Could you check a few things on this model? Use its own coordinates, in mm. A direction names the side the tool comes from. Coordinates: 2 decimals unless noted, no trailing zeros. Loops run counter-clockwise (first coordinate to the right, second up) from the corner with the lowest first, then second, coordinate; pieces in that order, holes last. Notation, with made-up numbers: (40.5, 14) -> (60.5, 14) arc R25 cw to (60.5, 47) -> close; hole circle Ø8 at (13.25, -19.5). An arc over 180 degrees is marked (long way). One line per question, with ' | ' between items. Start each with the question number.
(1) Suppose I cut it at A-A (y = -30.5). Please give me the cut outline in (x, z), plus the area to 3 significant figures.
(2) Which directions (+Z, -Z, +X, -X, +Y, -Y) give clear straight access to the entire face, cutting with the end or side of a thin tool? Please do faces 1 (the face through (33, -5, 2)), 2 (the face through (-28, 9, 2)), 3 (the face through (21.86, -19.44, 4.86)), 4 (the face through (20, 42.1, -1)), 5 (the face through (-32, 2, 0)).
(3) Suppose I cut it at C-C (z = -1). Please give me the cut outline in (x, y), plus the area to 3 significant figures.
(4) If we mould it in two halves opening along X, with no side actions, what happens to faces 6 (the face through (-30, -7, -2)), 7 (the face through (38.997, 0.154, 0.247)), 8 (the face through (28.1, -1, -1))? For each: pulls with the +X half, pulls with the -X half, needs draft (parallel to the pull), parting line crosses it, or undercut.
(5) I'm going to push flat-ended pins straight in: pin 1 Ø2.5 at (x, y) = (-35.5, 0) entering from +Z; pin 2 Ø1 at (y, z) = (40.5, 2.5) entering from +X; pin 3 Ø5 at (x, y) = (-36, 0.5) entering from -Z; pin 4 Ø11 at (x, y) = (-35.5, 0) entering from -Z. Where does each tip first touch, or does it pass through?
(6) If I drill on line 1 along X through (y, z) = (38.5, 1.95); line 2 along Y through (x, z) = (24.5, 3.5); line 3 along Y through (x, z) = (27, 3.75), over which ranges is the centre line in solid material (lowest first)?
(7) Suppose I cut it at D-D (y = 0). Give the number of separate pieces and of enclosed holes in the cut face, plus the area to 3 significant figures.
(8) Suppose I cut it at B-B (x = 6). Please give me the cut outline in (y, z).
```python
from build123d import *
from OCP.BRepFilletAPI import BRepFilletAPI_MakeChamfer

# Parameters (mm, degrees)
SKETCH1_R           = 0.85
BOSS_EXTRUDE1_DEPTH = 5
SKETCH2_W           = 56.2
SKETCH2_H           = 85.2
BOSS_EXTRUDE2_DEPTH = 2
SKETCH3_R           = 2.25
BOSS_EXTRUDE3_DEPTH = 5
SKETCH4_R           = 3.5
CUT_EXTRUDE1_DEPTH  = 3
SKETCH5_W           = 25
SKETCH5_H           = 2.4
CUT_EXTRUDE2_DEPTH  = 62.118736898
CHAMFER3_SIZE       = 0.5
CHAMFER1_SIZE       = 2.5
CHAMFER1_SIZE_2     = 1.25


with BuildPart() as part:
    # Sketch1 → Boss-Extrude1 (new body)
    with BuildSketch(Plane.XY):
        Polygon((-30.5, -43), (-30.5, 44.5), (30.5, 44.5), (30.5, -43), (30.5, -45.5), (-30.5, -45.5), align=None)
        with Locations((-24.5, 38.5)):
            Circle(SKETCH1_R, mode=Mode.SUBTRACT)
        with Locations((24.5, 38.5)):
            Circle(SKETCH1_R, mode=Mode.SUBTRACT)
        with Locations((24.5, -19.5)):
            Circle(SKETCH1_R, mode=Mode.SUBTRACT)
        with Locations((-24.5, -19.5)):
            Circle(SKETCH1_R, mode=Mode.SUBTRACT)
        with BuildLine():
            Line((-21.5, 38.5), (-21.5, 42))
            Line((-21.5, 42), (8, 42))
            Line((8, 42), (8, 35.5))
            Line((8, 35.5), (24.5, 35.5))
            Line((24.5, 35.5), (28, 35.5))
            Line((28, 35.5), (28, -16.5))
            Line((28, -16.5), (24.5, -16.5))
            ThreePointArc((24.5, -16.5), (21.5, -19.5), (24.5, -22.5))
            Line((24.5, -22.5), (28, -22.5))
            Line((28, -22.5), (28, -42))
            Line((28, -42), (5, -42))
            Line((5, -42), (5, -38))
            Line((5, -38), (0, -38))
            Line((0, -38), (-5, -38))
            Line((-5, -38), (-5, -42))
            Line((-5, -42), (-28, -42))
            Line((-28, -42), (-28, -22.5))
            Line((-28, -22.5), (-24.5, -22.5))
            ThreePointArc((-24.5, -22.5), (-21.5, -19.5), (-24.5, -16.5))
            Line((-24.5, -16.5), (-28, -16.5))
            Line((-28, -16.5), (-28, 35.5))
            Line((-28, 35.5), (-24.5, 35.5))
            ThreePointArc((-24.5, 35.5), (-22.378679656, 36.378679656), (-21.5, 38.5))
        make_face(mode=Mode.SUBTRACT)
    extrude(amount=BOSS_EXTRUDE1_DEPTH)

    # Sketch2 → Boss-Extrude2 (add)
    with BuildSketch(Plane.XY):
        Polygon((30.5, -45.5), (30.5, 44.5), (-30.5, 44.5), (-30.5, -45.5), (-28.1, -45.5), (28.1, -45.5), align=None)
        with Locations((0, -0.5)):
            Rectangle(SKETCH2_W, SKETCH2_H, mode=Mode.SUBTRACT)
    extrude(amount=-BOSS_EXTRUDE2_DEPTH)

    # Sketch3 → Boss-Extrude3 (add)
    # profile 1 of 2: a face of its own
    with BuildSketch(Plane.XY):
        with BuildLine():
            Line((35.5, 5), (30.5, 5))
            Line((30.5, 5), (30.5, -5))
            Line((30.5, -5), (35.5, -5))
            ThreePointArc((35.5, -5), (40.5, 0), (35.5, 5))
        make_face()
        with Locations(Location((35.5, 0, 0), (0, 0, 180))):
            Circle(SKETCH3_R, mode=Mode.SUBTRACT)
    # profile 2 of 2: a face of its own
    with BuildSketch(Plane.XY):
        with BuildLine():
            Line((-35.5, 5), (-30.5, 5))
            Line((-30.5, 5), (-30.5, -5))
            Line((-30.5, -5), (-35.5, -5))
            ThreePointArc((-35.5, -5), (-40.5, 0), (-35.5, 5))
        make_face()
        with Locations(Location((-35.5, 0, 0), (0, 0, 180))):
            Circle(SKETCH3_R, mode=Mode.SUBTRACT)
    extrude(amount=BOSS_EXTRUDE3_DEPTH)

    # Sketch4 → Cut-Extrude1 (cut)
    with BuildSketch(Plane(origin=(0, 0, 0), x_dir=(-1, 0, 0), z_dir=(0, 0, -1))):
        with Locations((-35.5, 0)):
            Circle(SKETCH4_R)
        with Locations((35.5, 0)):
            Circle(SKETCH4_R)
    extrude(amount=-CUT_EXTRUDE1_DEPTH, mode=Mode.SUBTRACT)

    # Sketch5 → Cut-Extrude2 (cut, through all)
    with BuildSketch(Plane(origin=(0, 0, 0), x_dir=(-1, 0, 0), z_dir=(0, 0, -1))):
        with Locations((0, 43.3)):
            Rectangle(SKETCH5_W, SKETCH5_H)
    extrude(amount=CUT_EXTRUDE2_DEPTH, mode=Mode.SUBTRACT)

    # Chamfer3
    chamfer3_edges = [part.edges().sort_by_distance(p)[0] for p in [
        (30.5, 44.5, 1.5),
        (30.5, -45.5, 1.5),
        (-30.5, -45.5, 1.5),
        (-30.5, 44.5, 1.5),
        (30.5, 24.75, 5),
        (40.5, 0, 5),
        (33, 5, 5),
        (33, -5, 5),
        (37.75, 0, 5),
        (-30.5, -25.25, 5),
        (-40.5, 0, 5),
        (-33, -5, 5),
        (-33, 5, 5),
        (-33.25, 0, 5),
        (0, -45.5, 5),
        (-25.35, 38.5, 0),
        (-25.35, 38.5, 5),
        (30.5, -25.25, 5),
        (23.65, 38.5, 0),
        (23.65, 38.5, 5),
        (-5, -38, 2.5),
        (5, -38, 2.5),
        (0, 44.5, 5),
        (8, 35.5, 2.5),
        (-22.378679656, 36.378679656, 5),
        (-26.25, 35.5, 5),
        (-28, 9.5, 5),
        (-26.25, -16.5, 5),
        (-21.5, -19.5, 5),
        (-26.25, -22.5, 5),
        (-28, -32.25, 5),
        (-16.5, -42, 5),
        (-5, -40, 5),
        (0, -38, 5),
        (5, -40, 5),
        (16.5, -42, 5),
        (28, -32.25, 5),
        (26.25, -22.5, 5),
        (21.5, -19.5, 5),
        (26.25, -16.5, 5),
        (28, 9.5, 5),
        (18, 35.5, 5),
        (8, 38.75, 5),
        (-6.75, 42, 5),
        (-21.5, 40.25, 5),
        (23.65, -19.5, 0),
        (23.65, -19.5, 5),
        (-25.35, -19.5, 0),
        (-25.35, -19.5, 5),
        (-30.5, 24.75, 5),
    ]]
    chamfer(chamfer3_edges, length=CHAMFER3_SIZE)

    # Chamfer1
    chamfer1_edges_1 = [part.edges().sort_by_distance(p)[0] for p in [
        (39, 0, 3),
    ]]
    chamfer1_side_1 = [part.faces().sort_by_distance(p)[0] for p in [
        (39, 0, 2.975),
    ]]
    chamfer1_edges_2 = [part.edges().sort_by_distance(p)[0] for p in [
        (-32, 0, 3),
    ]]
    chamfer1_side_2 = [part.faces().sort_by_distance(p)[0] for p in [
        (-32, 0, 2.975),
    ]]
    chamfer1 = BRepFilletAPI_MakeChamfer(part.part.solid().wrapped)
    for e in chamfer1_edges_1:
        chamfer1.Add(CHAMFER1_SIZE - 0.0001, CHAMFER1_SIZE_2 - 0.0001, e.wrapped, chamfer1_side_1[0].wrapped)
    for e in chamfer1_edges_2:
        chamfer1.Add(CHAMFER1_SIZE - 0.0001, CHAMFER1_SIZE_2 - 0.0001, e.wrapped, chamfer1_side_2[0].wrapped)
    add(Compound.cast(chamfer1.Shape()), mode=Mode.REPLACE)  # a hair under: the kernel refuses the full size


solid = part.part
```
Checks:
1) outline: (-30.5, -2) -> (-28.1, -2) -> (-28.1, 0) -> (-28, 0) -> (-28, 4.5) -> (-28.5, 5) -> (-30, 5) -> (-30.5, 4.5) -> close; (28, 0) -> (28.1, 0) -> (28.1, -2) -> (30.5, -2) -> (30.5, 4.5) -> (30, 5) -> (28.5, 5) -> (28, 4.5) -> close | area: 34.1 mm^2
2) face 1: +Z, -Z, +X, -Y | face 2: +Z, -Z | face 3: +Z | face 4: -Z | face 5: -Z, -X, +Y, -Y
3) outline: (-30.5, -45) -> (-30, -45.5) -> (30, -45.5) -> (30.5, -45) -> (30.5, 44) -> (30, 44.5) -> (12.5, 44.5) -> (12.5, 42.1) -> (28.1, 42.1) -> (28.1, -43.1) -> (-28.1, -43.1) -> (-28.1, 42.1) -> (-12.5, 42.1) -> (-12.5, 44.5) -> (-30, 44.5) -> (-30.5, 44) -> close | area: 641 mm^2
4) face 6: needs draft | face 7: undercut | face 8: undercut
5) pin 1: passes through | pin 2: stops at x = 30.5 | pin 3: stops at z = 1.09 | pin 4: stops at z = -2
6) line 1: x = -30.5 to -25.35, -23.65 to -21.5, 8 to 23.65, 25.35 to 30.5 | line 2: y = -45.5 to -42, -22.5 to -20.35, -18.65 to -16.5, 35.5 to 37.65, 39.35 to 44.5 | line 3: y = -45.5 to -42, -22.5 to -16.5, 35.5 to 44.5
7) separate pieces: 4 | enclosed holes: 0 | area: 79.8 mm^2
8) outline: (-45.5, -2) -> (-43.1, -2) -> (-43.1, 0) -> (-42, 0) -> (-42, 4.5) -> (-42.5, 5) -> (-45, 5) -> (-45.5, 4.5) -> close; (42, 0) -> (44.5, 0) -> (44.5, 4.5) -> (44, 5) -> (42.5, 5) -> (42, 4.5) -> close
